Check sheet for the drawn part. Datum: minimum x, y, z corner. Units: mm. Give positions to 0.01 mm unless a question says otherwise; leave off trailing zeros. Loops run counter-clockwise (first coordinate to the right, second up) from the corner with the lowest first, then second, coordinate; pieces in that order, holes last. Notation, with made-up numbers: (74, 40) - (130, 40) arc R16 ccw to (130, 54) - close; hole circle Ø1 at (4.25, 37.25). An arc over 180 degrees is marked (long way). Use a Markdown table: item, result. Add a question column.
1. Cross-section at B-B on y = 5.75. Enter the section's corners in (x, z) (3 decimals), and give its area (3 significant figures).
2. Depth check by flat-ended pin: P1, Ø4, axis at y = 6, z = 39.5, coming from the +X side; P2, Ø1.5, axis at x = 24.5, y = 2, coming from the +Z side; P3, Ø16, axis at x = 39.5, z = 39, coming from the +Y side; P4, Ø1, axis at x = 47, z = 47.5, coming from the +Y side. Enter the tip coordinate at first touch or a pass-through.
3. Material ranges on L1, parallel to Y at x = 14.5, z = 49.5; L2, parallel to X at y = 9.5, z = 28; L3, parallel to Z at x = 22, y = 1.5, recorded low to high.
4. Draft check along X on the marked faces 1, 2 and 3. Enter one of: pulls with the +X half, pulls with the -X half, needs draft (parallel to the pull), parting line crosses it, or undercut.
5. Cross-section at A-A on y = 13.25. Enter the section's corners in (x, z) (3 decimals).
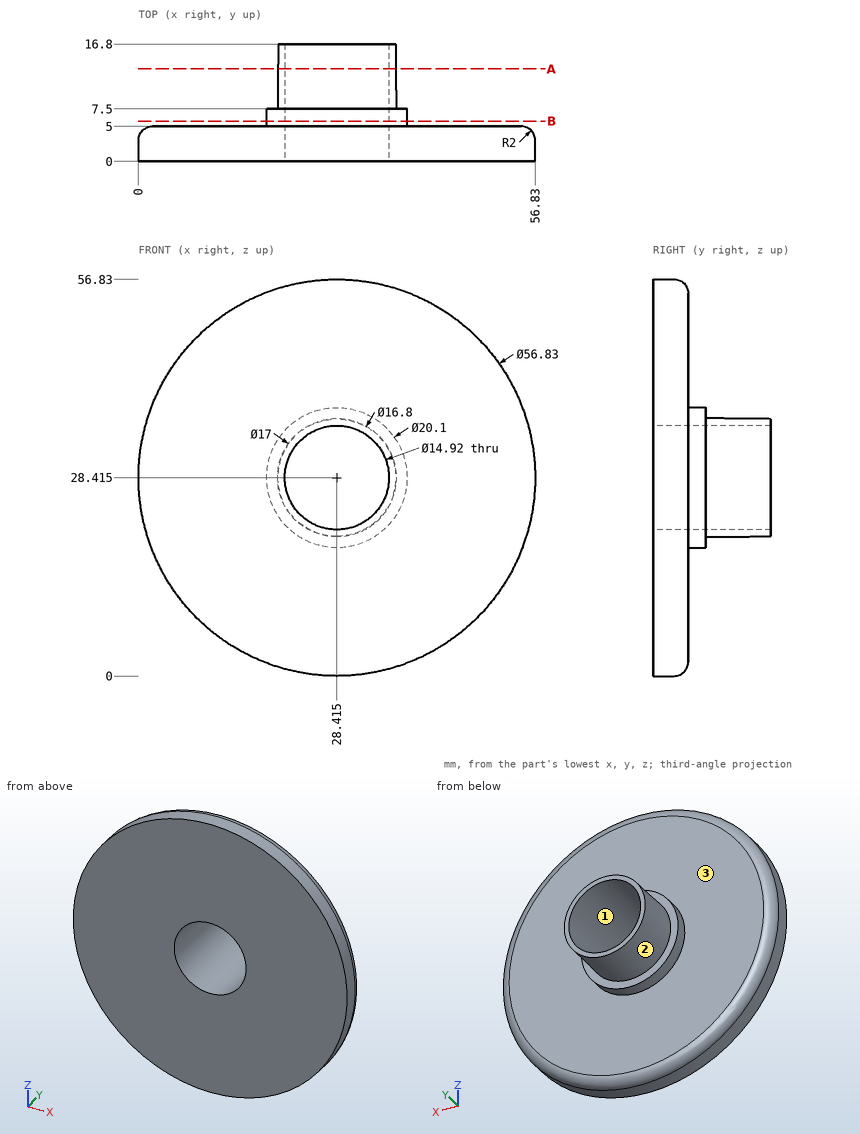
Values found:
| question | item | result |
|---|---|---|
| 1 | outline | circle Ø20.1 at (28.415, 28.415); hole circle Ø14.92 at (28.415, 28.415) |
| 1 | area | 142 mm2 |
| 2 | P1 | stops at x = 54.5 |
| 2 | P2 | stops at z = 56.65 |
| 2 | P3 | stops at y = 16.8 |
| 2 | P4 | stops at y = 5 |
| 3 | L1 | y = 0 to 5 |
| 3 | L2 | x = 19.95 to 20.97, 35.86 to 36.88 |
| 3 | L3 | z = 0.73 to 24.61, 32.22 to 56.1 |
| 4 | face 1 | undercut |
| 4 | face 2 | parting line crosses it |
| 4 | face 3 | needs draft |
| 5 | outline | circle Ø16.876 at (28.415, 28.415); hole circle Ø14.92 at (28.415, 28.415) |
